For this review, use the dimensioned drawing (mm, ordinates from the lowest corner) and the shaded views. Give positions to 0.01 mm unless a question says otherwise; leave off trailing zeros. Write each loop counter-clockwise with the first axis right and the second up, starting at its lowest first coordinate (ties: lowest second). Pieces come first, ordered by that corner, then holes.
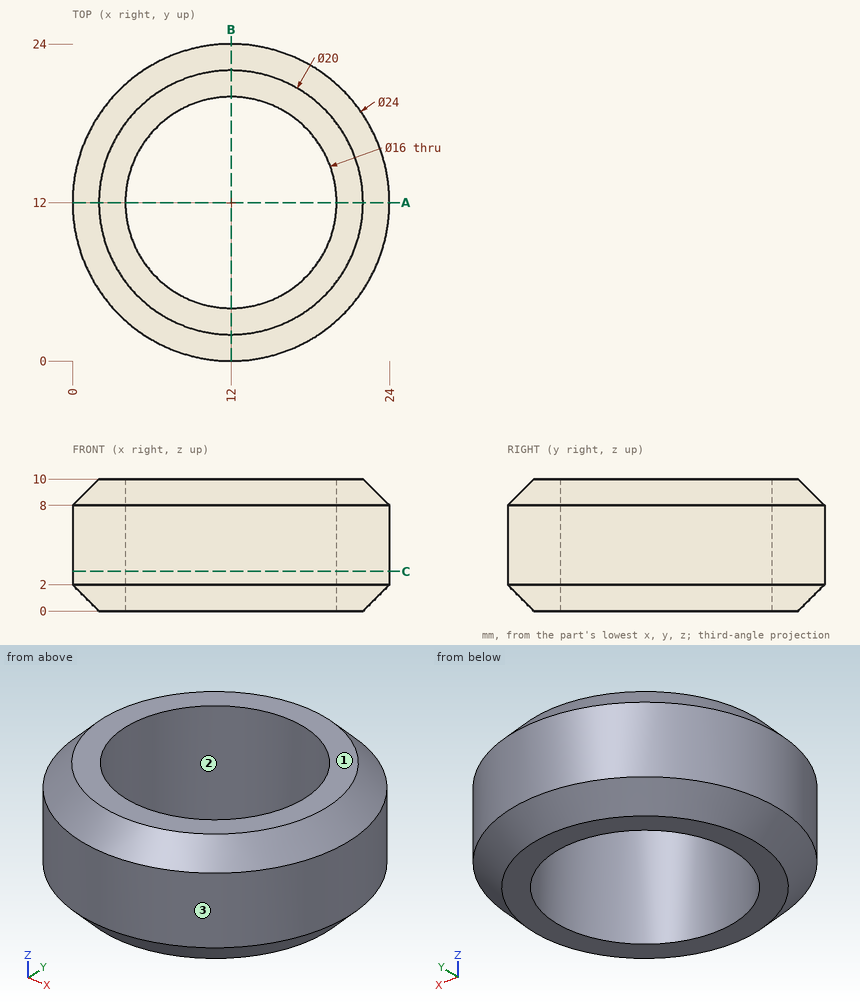
(1) The part is to be moulded in two halves that separate along X. For the marked faces 1, 2 and 3, say which applies: +X half, -X half, draft (parallel to the pull), parting line (faces both ways), or undercut.
(2) For L1, parallel to Y at x = 12, z = 2.5; L2, parallel to X at y = 8, z = 2.75; L3, parallel to X at y = 4.75, z = 1.75, list the stretches that pass through material, from the lowest coordinate up.
(3) Clearance check with flat-ended pins moving along their axes: pin 1 Ø9.5 at (x, y) = (12, 12) entering from -Z; pin 2 Ø1.5 at (y, z) = (18, 8.5) entering from -X; pin 3 Ø2 at (x, z) = (9.5, 7) entering from +Y; pin 4 Ø5 at (y, z) = (8, 8) entering from +X. State where each tip first meets the part, or that it passes through.
(4) We need section C-C (z = 3). Write out the cut boundary in (x, y).
(5) We need section A-A (y = 12). Write out the cut boundary in (x, z), and give its area (3 significant figures).
The answers:
1. face 1: draft
1. face 2: undercut
1. face 3: parting line
2. L1: y = 0 to 4, 20 to 24
2. L2: x = 0.69 to 5.07, 18.93 to 23.31
2. L3: x = 2.75 to 8.62, 15.38 to 21.25
3. pin 1: passes through
3. pin 2: stops at x = 1.3
3. pin 3: stops at y = 23.91
3. pin 4: stops at x = 23.91
4. outline: circle Ø24 at (12, 12); hole circle Ø16 at (12, 12)
5. outline: (0, 2) - (2, 0) - (4, 0) - (4, 10) - (2, 10) - (0, 8) - close; (20, 0) - (22, 0) - (24, 2) - (24, 8) - (22, 10) - (20, 10) - close
5. area: 72.0 mm2
